from build123d import *

# Parameters (mm, degrees)
F0_R     = 50
F0_R_2   = 24.99
F1_DEPTH = 50
F2_SIZE  = 5
F3_SIZE  = 5


with BuildPart() as f1:
    # F0 (on Top) → F1 (new body)
    with BuildSketch(Plane.XY):
        Circle(F0_R)
        Circle(F0_R_2, mode=Mode.SUBTRACT)
    extrude(amount=F1_DEPTH)

    # F2
    f2_edges = [f1.edges().sort_by_distance(p)[0] for p in [
        (-24.99, 0, 50),
    ]]
    chamfer(f2_edges, length=F2_SIZE)

    # F3
    f3_edges = [f1.edges().sort_by_distance(p)[0] for p in [
        (-50, 0, 0),
    ]]
    chamfer(f3_edges, length=F3_SIZE)


solid = f1.part
Read the model definition and answer for the solid it produces. Units are mm, in the model's axes. Give positions to 0.01 mm unless a question says otherwise; leave off trailing zeros. Loops run counter-clockwise (first coordinate to the right, second up) from the corner with the lowest first, then second, coordinate; pieces in that order, holes last. Notation, with made-up numbers: (8, 61) - (14, 61) arc R9 cw to (14, 69) - close; hole circle Ø3 at (53.5, 17). An arc over 180 degrees is marked (long way). Answer as CSV lines item,"result". Start each with the question number.
1) Determine the mould class of faces 1 (the face through (-5.49, -24.7, 45.31)), 2 (the face through (43.22, 13.61, 0.31)), 3 (the face through (19, -19, 0)) for opening direction Y: released by +Y, released by -Y, zero draft, split by the parting line, or undercut.
2) Find section A-A (y = 0). Write down the section's boundary in (x, z).
3) Find section C-C (z = 12). Write down the section's boundary in (x, y).
4) Each of these flat-tipped pins is pushed along its axis until it touches: pin 1 Ø8 at (y, z) = (13, 21) entering from +X; pin 2 Ø1.5 at (x, z) = (16, 30) entering from +Y; pin 3 Ø1.5 at (x, z) = (-7, 39.5) entering from +Y. Where does it stop, or does it pass through?
5) Straight lines are drawn through the part: L1, parallel to Y at x = 0, z = 27; L2, parallel to Y at x = -12, z = 3; L3, parallel to X at y = 4, z = 20.5. For each, find the intervals that lie inside material, in ascending order. Write a range as from..to.
Findings below:
1,face 1,"undercut"
1,face 2,"split by the parting line"
1,face 3,"zero draft"
2,outline,"(-50, 5) - (-45, 0) - (-24.99, 0) - (-24.99, 45) - (-29.99, 50) - (-50, 50) - close; (24.99, 0) - (45, 0) - (50, 5) - (50, 50) - (29.99, 50) - (24.99, 45) - close"
3,outline,"circle Ø100 at (0, 0); hole circle Ø49.98 at (0, 0)"
4,pin 1,"x = 49.18"
4,pin 2,"y = 47.62"
4,pin 3,"y = 49.61"
5,L1,"-50..-24.99, 24.99..50"
5,L2,"-46.48..-21.92, 21.92..46.48"
5,L3,"-49.84..-24.67, 24.67..49.84"
